For this review, take the finished solid that the model builds, in its own axes (mm). Face numbers are marked on the shaded views. A direction names the side the tool comes from. Give positions to 0.01 mm unless a question says otherwise; leave off trailing zeros. Order: outer loops, then holes, each group sorted by start corner. A loop starts at its lowest first (then second) coordinate and runs counter-clockwise, first axis right, second up.
from build123d import *

# Parameters (mm, degrees)
SKETCH1_R           = 2
BOSS_EXTRUDE1_DEPTH = 65
SKETCH2_R           = 4.5
BOSS_EXTRUDE2_DEPTH = 1
SKETCH3_R           = 2
SKETCH3_R_2         = 1.25
CUT_EXTRUDE1_DEPTH  = 6.4


with BuildPart() as part:
    # Sketch1 → Boss-Extrude1 (new body)
    with BuildSketch(Plane(origin=(0, 0, 0), x_dir=(0, 0, -1), z_dir=(1, 0, 0))):
        Circle(SKETCH1_R)
    extrude(amount=BOSS_EXTRUDE1_DEPTH)

    # Sketch2 → Boss-Extrude2 (add)
    with BuildSketch(Plane(origin=(13.4, 0, 0), x_dir=(0, 0, -1), z_dir=(1, 0, 0))):
        Circle(SKETCH2_R)
    extrude(amount=BOSS_EXTRUDE2_DEPTH)

    # Sketch3 → Cut-Extrude1 (cut)
    with BuildSketch(Plane(origin=(0, 0, 0), x_dir=(0, 0, -1), z_dir=(1, 0, 0))):
        Circle(SKETCH3_R)
        Circle(SKETCH3_R_2, mode=Mode.SUBTRACT)
    extrude(amount=CUT_EXTRUDE1_DEPTH, mode=Mode.SUBTRACT)


solid = part.part
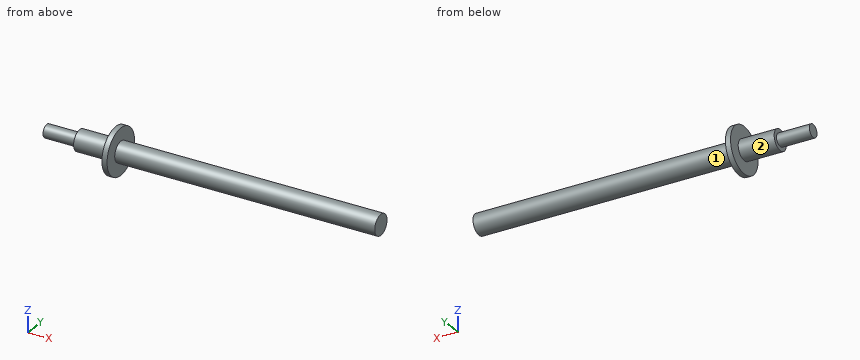
1) We need section D-D on y = 3.75. Give the boundary of the cut face in (x, z).
Answer sheet:
outline: (13.4, -2.49) - (14.4, -2.49) - (14.4, 2.49) - (13.4, 2.49) - close
2) Clearance check with flat-ended pins moving along their axes: pin 1 (3 mm diameter, centred on x = 32, z = 3, fed in from +Y); pin 2 (5 mm diameter, centred on x = 29, y = 1.5, fed in from +Z); pin 3 (1.5 mm diameter, centred on y = -1.5, z = 2.5, fed in from +X). State where each tip first meets the part, or that it passes through.
Answer sheet:
pin 1: stops at y = 1.32
pin 2: stops at z = 2
pin 3: stops at x = 14.4
3) To check wall thickness, follow line 1 (X direction, y = 2.25, z = -2.25); line 2 (Y direction, x = 3.5, z = -0.5); line 3 (Z direction, x = 25.5, y = 0.5). State the ranges of each line that lie inside material, in increasing order.
Answer sheet:
line 1: x = 13.4 to 14.4
line 2: y = -1.15 to 1.15
line 3: z = -1.94 to 1.94
4) Tool access review of the marked faces 1 and 2: name each direction out of +Z, -Z, +X, -X, +Y, -Y from which nothing blocks a thin tool from reaching the whole face with its end or side.
Answer sheet:
face 1: +X
face 2: -X
5) We need section A-A on z = 0. Give the boundary of the cut face in (x, y), then the cut area to 3 significant figures.
Answer sheet:
outline: (0, -1.25) - (6.4, -1.25) - (6.4, -2) - (13.4, -2) - (13.4, -4.5) - (14.4, -4.5) - (14.4, -2) - (65, -2) - (65, 2) - (14.4, 2) - (14.4, 4.5) - (13.4, 4.5) - (13.4, 2) - (6.4, 2) - (6.4, 1.25) - (0, 1.25) - close
area: 255 mm2
6) We need section C-C on x = 60.5. Give the boundary of the cut face in (y, z), then the cut area to 3 significant figures.
Answer sheet:
outline: circle Ø4 at (0, 0)
area: 12.6 mm2
